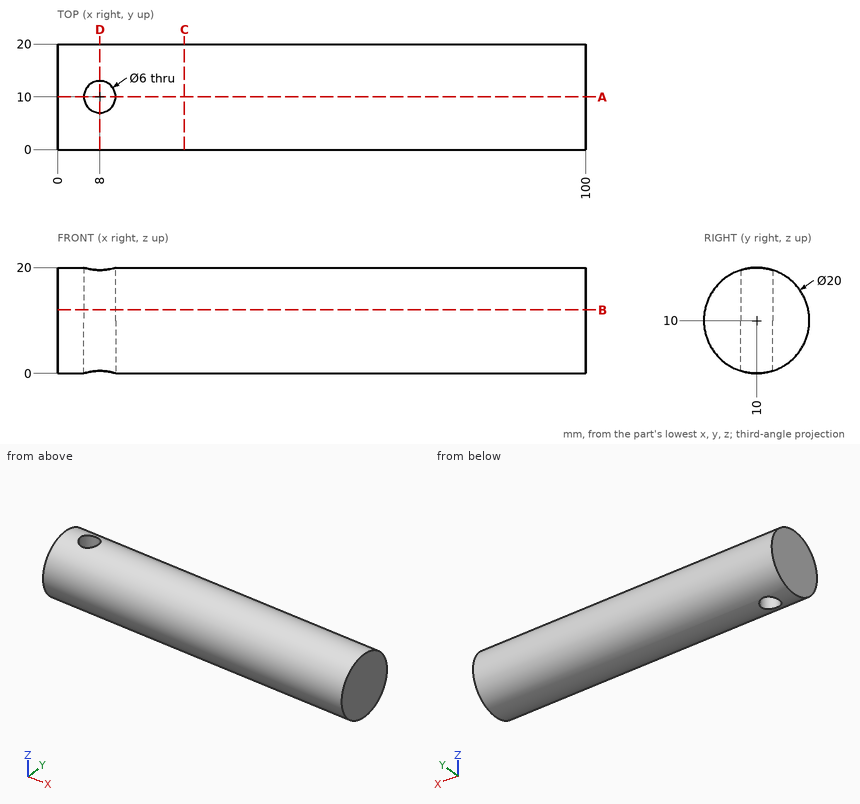
Geometry check sheet. Reference: drawing and pictorial views, mm from the part's lowest x, y, z. Give positions to 0.01 mm unless a question says otherwise; leave off trailing zeros. Order: outer loops, then holes, each group sorted by start corner. A loop starts at its lowest first (then second) coordinate and runs counter-clockwise, first axis right, second up. Notation, with made-up numbers: (75.25, 29.25) - (97.25, 29.25) arc R15 ccw to (97.25, 41.25) - close; hole circle Ø6 at (58, -10). An arc over 180 degrees is marked (long way). Answer as CSV lines item,"result".
1. Section check A-A (y = 10). Record the boundary of the cut face in (x, z), then the cut area to 3 significant figures.
Result sheet:
outline,"(0, 0) - (5, 0) - (5, 20) - (0, 20) - close; (11, 0) - (100, 0) - (100, 20) - (11, 20) - close"
area,"1,880 mm²"
2. Go/stop test with flat-tipped pins: P1, Ø2, axis at x = 16.5, y = 16, coming from the -Z side; P2, Ø1.5, axis at x = 71, z = 12, coming from the -Y side; P3, Ø8, axis at x = 8, y = 10, coming from the -Z side; P4, Ø1, axis at x = 56.5, z = 16.5, coming from the +Y side. Record where each tip stops, or that it passes through.
Result sheet:
P1,"z = 1.34"
P2,"y = 0.08"
P3,"z = 0"
P4,"y = 18"
3. Section check B-B (z = 12). Record the boundary of the cut face in (x, y), then the cut area to 3 significant figures.
Result sheet:
outline,"(0, 0.2) - (100, 0.2) - (100, 19.8) - (0, 19.8) - close; hole circle Ø6 at (8, 10)"
area,"1,930 mm²"
4. Scan lines: probe 1 along Z at (x, y) = (67.5, 10.5); probe 2 along X at (y, z) = (9.25, 4.25); probe 3 along X at (y, z) = (11.75, 9.25). Record each from-to range of solid material in increasing order. Write a range as from..to.
Result sheet:
probe 1,"0.01..19.99"
probe 2,"0..5.1, 10.9..100"
probe 3,"0..5.56, 10.44..100"
5. Section check D-D (x = 8). Record the boundary of the cut face in (y, z), then the cut area to 3 significant figures.
Result sheet:
outline,"(7, 0.46) - (7, 19.54) arc R10 ccw to start; (13, 0.46) arc R10 ccw to (13, 19.54) - close"
area,"196 mm²"
6. Section check C-C (x = 24). Record the boundary of the cut face in (y, z), then the cut area to 3 significant figures.
Result sheet:
outline,"circle Ø20 at (10, 10)"
area,"314 mm²"
